Source: CAD feature listing. Evaluate the final solid. Frame: model axes, mm. A direction names the side the tool comes from. Coordinates: 2 decimals unless noted, no trailing zeros. Loops run counter-clockwise (first coordinate to the right, second up) from the corner with the lowest first, then second, coordinate; pieces in that order, holes last.
```python
from build123d import *

# Parameters (mm, degrees)
SKETCH1_R           = 0.634780864
BOSS_EXTRUDE1_DEPTH = 1.65
FILLET1_R           = 0.7112
FILLET2_R           = 0.7112
FILLET3_R           = 1.27


with BuildPart() as part:
    # Sketch1 → Boss-Extrude1 (new body)
    with BuildSketch(Plane.XY):
        with BuildLine():
            Line((-27.135222714, 29.397964527), (-29.397964527, 27.135222714))
            Line((-29.397964527, 27.135222714), (-21.855060774, 19.592318961))
            ThreePointArc((-21.855060774, 19.592318961), (-15.928204538, 10.7930358), (-13.742710724, 0.41138729))
            Line((-13.742710724, 0.41138729), (-15.908512943, 0.41138729))
            Line((-15.908512943, 0.41138729), (-15.908512943, -0.41138729))
            Line((-15.908512943, -0.41138729), (-13.742710724, -0.41138729))
            ThreePointArc((-13.742710724, -0.41138729), (-15.928204538, -10.7930358), (-21.855060774, -19.592318961))
            Line((-21.855060774, -19.592318961), (-29.397964527, -27.135222714))
            Line((-29.397964527, -27.135222714), (-27.135222714, -29.397964527))
            Line((-27.135222714, -29.397964527), (-19.592318961, -21.855060774))
            ThreePointArc((-19.592318961, -21.855060774), (-10.842511416, -15.949186255), (-0.51885361, -13.744514983))
            ThreePointArc((-0.51885361, -13.744514983), (0, -15.324082887), (0.51885361, -13.744514983))
            ThreePointArc((0.51885361, -13.744514983), (10.842511416, -15.949186255), (19.592318961, -21.855060774))
            Line((19.592318961, -21.855060774), (27.135222714, -29.397964527))
            Line((27.135222714, -29.397964527), (29.397964527, -27.135222714))
            Line((29.397964527, -27.135222714), (21.855060774, -19.592318961))
            ThreePointArc((21.855060774, -19.592318961), (17.437236913, -13.828628501), (14.668755804, -7.114999994))
            Line((14.668755804, -7.114999994), (15.618947426, -7.114999994))
            Line((15.618947426, -7.114999994), (15.618947426, 7.114999994))
            Line((15.618947426, 7.114999994), (14.668755804, 7.114999994))
            ThreePointArc((14.668755804, 7.114999994), (17.437236913, 13.828628501), (21.855060774, 19.592318961))
            Line((21.855060774, 19.592318961), (29.397964527, 27.135222714))
            Line((29.397964527, 27.135222714), (27.135222714, 29.397964527))
            Line((27.135222714, 29.397964527), (19.592318961, 21.855060774))
            ThreePointArc((19.592318961, 21.855060774), (10.842511416, 15.949186255), (0.51885361, 13.744514983))
            ThreePointArc((0.51885361, 13.744514983), (0, 15.324082887), (-0.51885361, 13.744514983))
            ThreePointArc((-0.51885361, 13.744514983), (-10.842511416, 15.949186255), (-19.592318961, 21.855060774))
            Line((-19.592318961, 21.855060774), (-27.135222714, 29.397964527))
        make_face()
        with Locations((0, 14.449082887)):
            Circle(SKETCH1_R, mode=Mode.SUBTRACT)
        with Locations((0, -14.449082887)):
            Circle(SKETCH1_R, mode=Mode.SUBTRACT)
    extrude(amount=BOSS_EXTRUDE1_DEPTH)

    # Fillet1
    fillet1_edges = [part.edges().sort_by_distance(p)[0] for p in [
        (0.51885361, 13.744514983, 0.825),
        (0.51885361, -13.744514983, 0.825),
        (-0.51885361, -13.744514983, 0.825),
        (-0.51885361, 13.744514983, 0.825),
    ]]
    fillet(fillet1_edges, radius=FILLET1_R)

    # Fillet2
    fillet2_edges = [part.edges().sort_by_distance(p)[0] for p in [
        (14.668755804, 7.114999994, 0.825),
        (14.668755804, -7.114999994, 0.825),
    ]]
    fillet(fillet2_edges, radius=FILLET2_R)

    # Fillet3
    fillet3_edges = [part.edges().sort_by_distance(p)[0] for p in [
        (-13.742710724, -0.41138729, 0.825),
        (-13.742710724, 0.41138729, 0.825),
    ]]
    fillet(fillet3_edges, radius=FILLET3_R)


solid = part.part
```
Q1. Draft query along X for faces 1 (the flat face through (25.68, -23.42, 0.81)), 2 (the flat face through (0, 0, 0)), 3 (the flat face through (23.31, -25.57, 0.81)), 4 (the flat face through (-28.282, -28.251, 0.813)). Return one class per face: released by +X, released by -X, zero draft, split by the parting line, or undercut.
Q2. Section query A-A on y = -16. Return the cut outline in (x, z), then the cut area to 3 significant figures.
Q3. Section query D-D on z = 1.1. Count the separate pieces of the cut face and the enclosed holes in it, then the cut area to 3 significant figures.
Q4. Reachability of faces 5 (the flat face through (28.251, -28.282, 0.813)), 6 (the flat face through (-23.42, -25.68, 0.81)), 7 (the cylindrical face through (-16.14, -11.28, 0.81)), 8 (the flat face through (-23.31, 25.57, 0.81)), 9 (the flat face through (15.619, 0, 1)) from +Z, -Z, +X, -X, +Y, -Y: full face, straight path, thin tool, end or side. Return the list, or none.
Q5. Material intervals for line 1 along Y through (x, z) = (0, 1.2); line 2 along Y through (x, z) = (-18, 0.8); line 3 along Y through (x, z) = (-22, 0.35), sorted ascending.
Q6. Section query C-C on y = 4. Return the cut outline in (x, z).
Q7. First-contact query: pin 1 Ø0.7 at (x, z) = (-15.5, 1) entering from +Y; pin 2 Ø1 at (x, y) = (0, -14.45) entering from +Z (3 decimals); pin 3 Ø0.5 at (y, z) = (2.5, 0.5) entering from +X. Flat tips, straight axial feed; report the tip coordinate or a pass-through.
Q8. Section query B-B on x = -23. Return the cut outline in (y, z), then the cut area to 3 significant figures.
Resolved:
1. face 1: released by +X
1. face 2: zero draft
1. face 3: undercut
1. face 4: released by -X
2. outline: (-18.83, 0) - (-10.96, 0) - (-10.96, 1.65) - (-18.83, 1.65) - close; (10.96, 0) - (18.83, 0) - (18.83, 1.65) - (10.96, 1.65) - close
2. area: 26.0 mm2
3. separate pieces: 1
3. enclosed holes: 2
3. area: 1,190 mm2
4. face 5: +Z, -Z, +X, -Y
4. face 6: +Z, -Z, -Y
4. face 7: +Z, -Z, -X
4. face 8: +Z, -Z, +Y
4. face 9: +Z, -Z, +X
5. line 1: y = -15.32 to -15.08, -13.81 to 13.81, 15.08 to 15.32
5. line 2: y = -20.38 to -14.76, 14.76 to 20.38
5. line 3: y = -24.26 to -19.74, 19.74 to 24.26
6. outline: (-14.03, 0) - (15.62, 0) - (15.62, 1.65) - (-14.03, 1.65) - close
7. pin 1: stops at y = 18.72
7. pin 2: passes through
7. pin 3: stops at x = 15.62
8. outline: (-25.26, 0) - (-20.74, 0) - (-20.74, 1.65) - (-25.26, 1.65) - close; (20.74, 0) - (25.26, 0) - (25.26, 1.65) - (20.74, 1.65) - close
8. area: 14.9 mm2
